Input: dimensioned drawing with shaded views. Units: mm. Origin: part minimum x, y, z. A direction names the side the tool comes from. Coordinates: 2 decimals unless noted, no trailing zeros. Order: outer loops, then holes, each group sorted by start corner. A loop starts at its lowest first (then second) coordinate and runs counter-clockwise, first axis right, second up. Notation, with made-up numbers: M -12.5,-34 L 33.5,-34 A22 cw 33.5,-17 Z; hole C -32,-24 d9. An arc over 180 degrees is marked long. Write item = value, one per line.
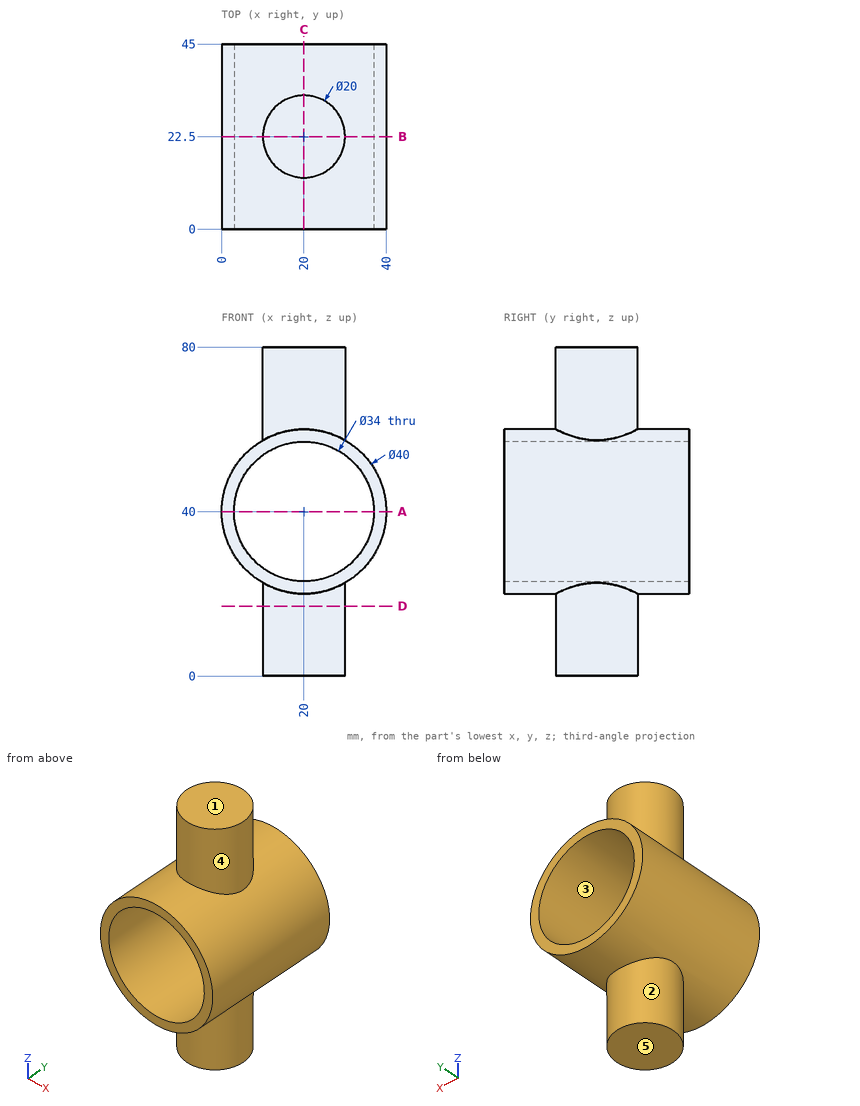
1) Section D-D, the plane z = 17. Return loops of the section in (x, y).
Numbers:
outline = C 20,22.5 d20
2) Section C-C, the plane x = 20. Return loops of the section in (y, z).
Numbers:
outline = M 0,20 L 12.5,20 L 12.5,0 L 32.5,0 L 32.5,20 L 45,20 L 45,23 L 0,23 Z; M 0,57 L 45,57 L 45,60 L 32.5,60 L 32.5,80 L 12.5,80 L 12.5,60 L 0,60 Z
3) Section A-A, the plane z = 40. Return loops of the section in (x, y).
Numbers:
outline = M 0,0 L 3,0 L 3,45 L 0,45 Z; M 37,0 L 40,0 L 40,45 L 37,45 Z
4) Section B-B, the plane y = 22.5. Return loops of the section in (x, z), and give its area (3 significant figures).
Numbers:
outline = M 10,0 L 30,0 L 30,22.68 A20 ccw 30,57.32 L 30,80 L 10,80 L 10,57.32 A20 ccw 10,22.68 Z; hole C 20,40 d34
area = 1,180 mm²
5) Pin query (flat end, axial travel): pin 1 (6 mm diameter, centred on x = 26.5, z = 64, fed in from +Y); pin 2 (10 mm diameter, centred on y = 5.5, z = 24, fed in from +X). Return the tip coordinate at first contact, or that it passes through.
Numbers:
pin_1 = 31.87
pin_2 = 36.7
6) Mould query, pull axis X, two halves, no side actions, for the marked faces 3, 4 and 5. Classes: pulls with the +X half, pulls with the -X half, needs draft (parallel to the pull), parting line crosses it, or undercut.
Numbers:
face_3 = undercut
face_4 = parting line crosses it
face_5 = needs draft
7) Line query: L1, parallel to X at y = 34.5, z = 40; L2, parallel to Z at x = 22.5, y = 10; L3, parallel to X at y = 33, z = 32. Output: solid intervals per line, ascending.
Numbers:
L1 = 0 to 3, 37 to 40
L2 = 20.16 to 23.18, 56.82 to 59.84
L3 = 1.67 to 5, 35 to 38.33
8) Set-up query: the marked faces 1 and 2. Return all of +Z, -Z, +X, -X, +Y, -Y with unobstructed straight access to the full face (end or side cutting, diameter ignored); none if empty.
Numbers:
face_1 = +Z, +X, -X, +Y, -Y
face_2 = -Z
